CAD build for the part. Positions are in the model's coordinates, mm. A direction names the side the tool comes from. Round coordinates to 2 decimals unless told otherwise and drop trailing zeros. Order: outer loops, then holes, each group sorted by start corner. A loop starts at its lowest first (then second) coordinate and runs counter-clockwise, first axis right, second up. Notation, with made-up numbers: M -5.5,47 L 32.5,47 A34 cw 32.5,83 Z; hole C 30,-22 d10. An arc over 180 degrees is marked long. Answer as a JSON object with one key per item and string values.
Autodesk Fusion 360 part; units mm, degrees
sketch "Sketch1" plane through (0, 0, 0) normal (0, 0, 1) x (1, 0, 0)
  line L0 (-50, 50) -> (200, 50)
  line L1 (200, 50) -> (200, -150)
  line L2 (200, -150) -> (-50, -150)
  line L3 (-50, -150) -> (-50, 50)
  line L4 (-55, 25) -> (-55, 51)
  line L5 (-55, 55) -> (-25, 55)
  line L6 (-51, 55) -> (201, 55)
  line L7 (205, 51) -> (205, -151)
  line L8 (201, -155) -> (-51, -155)
  line L9 (-55, -151) -> (-55, 55)
  arc A0 (-51, 55) -> (-55, 51) centre (-51, 51) ccw
  arc A1 (205, 51) -> (201, 55) centre (201, 51) ccw
  arc A2 (201, -155) -> (205, -151) centre (201, -151) ccw
  arc A3 (-55, -151) -> (-51, -155) centre (-51, -151) ccw
  point P0 (205, 55)
  point P1 (-55, -155)
  dimension "d1" = 250
  dimension "d2" = 200
  dimension "d3" = 260
  dimension "d4" = 210
  dimension "d5" = 4
  dimension "d6" = 4
  dimension "d7" = 4
  dimension "d8" = 4
extrude "Extrude1" add sketch "Sketch1" along normal blind 50 contours L4 L5 L6 L7 L8 L9 A0 A1 A2 A3
sketch "Sketch2" plane through (0, 0, 0) normal (0, 0, -1) x (1, 0, 0)
  line L0 (-50, 150) -> (200, 150)
  line L1 (200, 150) -> (200, -50)
  line L2 (200, -50) -> (-50, -50)
  line L3 (-50, -50) -> (-50, 150)
  line L4 (-55, 151) -> (-55, -51)
  arc A0 (-55, -51) -> (-51, -55) centre (-51, -51) ccw
  line L5 (-51, -55) -> (201, -55)
  arc A1 (201, -55) -> (205, -51) centre (201, -51) ccw
  line L6 (205, -51) -> (205, 151)
  arc A2 (205, 151) -> (201, 155) centre (201, 151) ccw
  line L7 (201, 155) -> (-51, 155)
  arc A3 (-51, 155) -> (-55, 151) centre (-51, 151) ccw
sketch "Sketch3" plane through (0, 0, 0) normal (0, 0, -1) x (1, 0, 0)
  line L0 (-51, 155) -> (201, 155)
  line L1 (205, 151) -> (205, -51)
  line L2 (201, -55) -> (-51, -55)
  line L3 (-55, -51) -> (-55, 151)
  arc A0 (201, -55) -> (205, -51) centre (201, -51) ccw
  arc A1 (205, 151) -> (201, 155) centre (201, 151) ccw
  arc A2 (-51, 155) -> (-55, 151) centre (-51, 151) ccw
  arc A3 (-55, -51) -> (-51, -55) centre (-51, -51) ccw
  dimension "d11" = 4
  dimension "d12" = 4
  dimension "d13" = 4
  dimension "d14" = 4
extrude "Extrude2" add sketch "Sketch3" along normal blind 5
sketch "Sketch4" plane through (0, 0, 50) normal (0, 0, 1) x (-1, 0, 0)
  line L0 (-200, 150) -> (50, 150)
  line L1 (50, 150) -> (50, -50)
  line L2 (50, -50) -> (-200, -50)
  line L3 (-200, -50) -> (-200, 150)
  line L4 (55, -51) -> (55, 151)
  arc A0 (55, 151) -> (51, 155) centre (51, 151) ccw
  line L5 (51, 155) -> (-201, 155)
  arc A1 (-201, 155) -> (-205, 151) centre (-201, 151) ccw
  line L6 (-205, 151) -> (-205, -51)
  arc A2 (-205, -51) -> (-201, -55) centre (-201, -51) ccw
  line L7 (-201, -55) -> (51, -55)
  arc A3 (51, -55) -> (55, -51) centre (51, -51) ccw
  circle A4 centre (52, -52) radius 2
  circle A5 centre (-202, -52) radius 2
  circle A6 centre (-202, 152) radius 2
  circle A7 centre (52, 152) radius 2
  dimension "d17" = 4
  dimension "d18" = 4
  dimension "d19" = 4
extrude "Extrude3" cut sketch "Sketch4" against normal blind 10 contours A4 | A5 | A6 | A7
thread "Thread1" thread offset 0 thread length 10
thread "Thread2" thread offset 0 thread length 10
Item 1: Saw through at A-A on z = 10.5. List the corners of the cut face in (x, y), and give its area (3 significant figures).
Worked answers:
{"outline": "M -55,-151 A4 ccw -51,-155 L 201,-155 A4 ccw 205,-151 L 205,51 A4 ccw 201,55 L -51,55 A4 ccw -55,51 Z; hole M -50,-150 L 200,-150 L 200,50 L -50,50 Z", "area": "4,590 mm2"}
Item 2: Wall check: line 1 along X through (y, z) = (38, 29.5); line 2 along Y through (x, z) = (170, 7); line 3 along Y through (x, z) = (-52, 44). Give the ranges that are in metal, low to high. Write a range as [from, to].
Worked answers:
{"line 1": "x = [-55, -50], [200, 205]", "line 2": "y = [-155, -150], [50, 55]", "line 3": "y = [-154.87, -154], [-150, 50], [54, 54.87]"}
Item 3: Drop flat-ended pins along their axis: pin 1 Ø6 at (x, y) = (169.5, -22) entering from +Z; pin 2 Ø1.2 at (x, y) = (-51.5, 52) entering from +Z. Give the stop position or say it passes through.
Worked answers:
{"pin 1": "stops at z = 0", "pin 2": "stops at z = 40"}
Item 4: 3-axis set-ups, long thin cutter, end or side, ignore diameter. For faces 1 (the flat face through (-51, -50, 50)), 2 (the flat face through (73, -51, 0)): which of +Z, -Z, +X, -X, +Y, -Y reach the whole face in a straight line?
Worked answers:
{"face 1": "+Z, +X, -X, +Y, -Y", "face 2": "+Z"}
Item 5: Saw through at C-C on x = 145.5. List the corners of the cut face in (y, z).
Worked answers:
{"outline": "M -155,-5 L 55,-5 L 55,50 L 50,50 L 50,0 L -150,0 L -150,50 L -155,50 Z"}
Item 6: Two-plate mould, pull along Y, no slides. Class faces 3 (the flat face through (73, -51, -5)), 4 (the flat face through (77, -150, 25)), 5 (the flat face through (77, -155, 22)): released by +Y, released by -Y, zero draft, split by the parting line, or undercut.
Worked answers:
{"face 3": "zero draft", "face 4": "undercut", "face 5": "released by -Y"}
Item 7: Saw through at B-B on y = -38.5. List the corners of the cut face in (x, z), and give its area (3 significant figures).
Worked answers:
{"outline": "M -55,-5 L 205,-5 L 205,50 L 200,50 L 200,0 L -50,0 L -50,50 L -55,50 Z", "area": "1,800 mm2"}
